Geometry: final body of the model. Coordinates: model frame, mm. Face numbers are marked on the shaded views. A direction names the side the tool comes from. Give positions to 0.01 mm unless a question says otherwise; leave off trailing zeros. Order: outer loops, then holes, each group sorted by start corner. A loop starts at its lowest first (then second) coordinate and runs counter-clockwise, first axis right, second up. Notation, with made-up numbers: (-38, 46.5) -> (21, 46.5) arc R15 cw to (21, 55.5) -> close; hole circle Ø1 at (76, 51.25). An arc over 180 degrees is marked (long way). Write item = value, one per line.
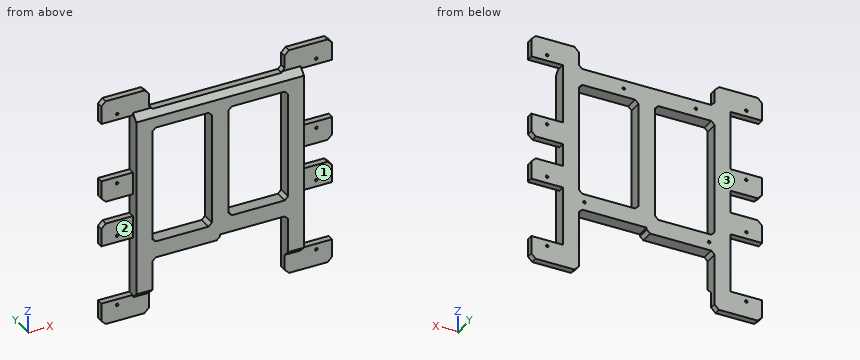
```python
from build123d import *

# Parameters (mm, degrees)
SKETCH1_W               = 89.4
SKETCH1_H               = 89.4
SKETCH1_R               = 0.5
BOSS_EXTRUDE1_DEPTH     = 2.5
SKETCH5_W               = 65
SKETCH5_H               = 74
BOSS_EXTRUDE3_DEPTH     = 2.5
SKETCH7_R               = 0.5
CUT_EXTRUDE2_DEPTH      = 4
CUT_EXTRUDE1_DEPTH      = 64.412774738
CUT_EXTRUDE1_DEPTH_BACK = 64.412774738
SKETCH2_W               = 12.2
SKETCH2_H               = 23
SKETCH2_W_2             = 52.6
SKETCH2_H_2             = 8.025
SKETCH2_W_3             = 23.1
SKETCH2_H_3             = 45.67
SKETCH2_H_4             = 43.68
SKETCH2_H_5             = 8.8
CHAMFER2_SIZE           = 1.3
CHAMFER3_SIZE           = 1.3
CHAMFER4_SIZE           = 1.7
CHAMFER5_SIZE           = 2.5


with BuildPart() as part:
    # Sketch1 → Boss-Extrude1 (new body)
    with BuildSketch(Plane(origin=(0, 0, 0), x_dir=(1, 0, 0), z_dir=(0, 1, 0))):
        Rectangle(SKETCH1_W, SKETCH1_H)
        with Locations(Location((-38.6, 38.3, 0), (0, 0, 270))):
            Circle(SKETCH1_R, mode=Mode.SUBTRACT)
        with Locations(Location((-38.6, 10.5, 0), (0, 0, 270))):
            Circle(SKETCH1_R, mode=Mode.SUBTRACT)
        with Locations(Location((-38.6, -10.5, 0), (0, 0, 270))):
            Circle(SKETCH1_R, mode=Mode.SUBTRACT)
        with Locations(Location((-38.6, -38.3, 0), (0, 0, 270))):
            Circle(SKETCH1_R, mode=Mode.SUBTRACT)
        with Locations(Location((38.6, -38.3, 0), (0, 0, 90))):
            Circle(SKETCH1_R, mode=Mode.SUBTRACT)
        with Locations(Location((38.6, -10.5, 0), (0, 0, 90))):
            Circle(SKETCH1_R, mode=Mode.SUBTRACT)
        with Locations(Location((38.6, 10.5, 0), (0, 0, 90))):
            Circle(SKETCH1_R, mode=Mode.SUBTRACT)
        with Locations(Location((38.6, 38.3, 0), (0, 0, 90))):
            Circle(SKETCH1_R, mode=Mode.SUBTRACT)
    extrude(amount=BOSS_EXTRUDE1_DEPTH)

    # Sketch5 → Boss-Extrude3 (add)
    with BuildSketch(Plane.XZ):
        Rectangle(SKETCH5_W, SKETCH5_H)
    extrude(amount=BOSS_EXTRUDE3_DEPTH)

    # Sketch7 → Cut-Extrude2 (cut)
    with BuildSketch(Plane(origin=(0, 2.5, 0), x_dir=(1, 0, 0), z_dir=(0, 1, 0))):
        with Locations(Location((-24.15, 18.595, 0), (0, 0, 270))):
            Circle(SKETCH7_R)
        with Locations(Location((24.15, 16.605, 0), (0, 0, 270))):
            Circle(SKETCH7_R)
        with Locations(Location((-19.07, -33.475, 0), (0, 0, 270))):
            Circle(SKETCH7_R)
        with Locations(Location((8.86, -33.475, 0), (0, 0, 270))):
            Circle(SKETCH7_R)
    extrude(amount=-CUT_EXTRUDE2_DEPTH, mode=Mode.SUBTRACT)

    # Sketch2 → Cut-Extrude1 (cut, two sides: drawn at the far end of the back side and taken through both)
    with BuildSketch(Plane(origin=(0, 2.5, 0), x_dir=(1, 0, 0), z_dir=(0, 1, 0)).offset(-CUT_EXTRUDE1_DEPTH_BACK)):
        with Locations((-38.6, 24.55)):
            Rectangle(SKETCH2_W, SKETCH2_H)
        Polygon((-26.3, 44.7), (26.3, 44.7), (26.3, 24.23), (26.3, 19.805), (0, 19.805), (0, 21.795), (-26.3, 21.795), align=None)
        with Locations((0, -40.6875)):
            Rectangle(SKETCH2_W_2, SKETCH2_H_2)
        with Locations((-14.75, -7.44)):
            Rectangle(SKETCH2_W_3, SKETCH2_H_3)
        with Locations((14.75, -8.435)):
            Rectangle(SKETCH2_W_3, SKETCH2_H_4)
        with Locations((-38.6, 0)):
            Rectangle(SKETCH2_W, SKETCH2_H_5)
        with Locations((38.6, 0)):
            Rectangle(SKETCH2_W, SKETCH2_H_5)
        with Locations((38.6, 24.55)):
            Rectangle(SKETCH2_W, SKETCH2_H)
        with Locations((38.6, -24.55)):
            Rectangle(SKETCH2_W, SKETCH2_H)
        with Locations((-38.6, -24.55)):
            Rectangle(SKETCH2_W, SKETCH2_H)
    extrude(amount=CUT_EXTRUDE1_DEPTH + CUT_EXTRUDE1_DEPTH_BACK, mode=Mode.SUBTRACT)

    # Chamfer2
    chamfer2_edges = [part.edges().sort_by_distance(p)[0] for p in [
        (0, 0, -21.795),
    ]]
    chamfer(chamfer2_edges, length=CHAMFER2_SIZE)

    # Chamfer3
    chamfer3_edges = [part.edges().sort_by_distance(p)[0] for p in [
        (-26.3, 0, -21.795),
        (26.3, 0, 36.675),
        (-26.3, 0, 36.675),
        (-26.3, 0, 30.275),
        (-3.2, 0, 30.275),
        (3.2, 0, 30.275),
        (26.3, 0, 30.275),
        (-3.2, 0, -15.395),
        (3.2, 0, -13.405),
        (26.3, 0, -13.405),
        (26.3, 0, -19.805),
        (-26.3, 0, -15.395),
    ]]
    chamfer(chamfer3_edges, length=CHAMFER3_SIZE)

    # Chamfer4
    chamfer4_edges = [part.edges().sort_by_distance(p)[0] for p in [
        (26.3, 1.25, 44.7),
        (-26.3, 1.25, 44.7),
        (-44.7, 1.25, 4.4),
        (-44.7, 1.25, -4.4),
        (-26.3, 1.25, -44.7),
        (26.3, 1.25, -44.7),
        (44.7, 1.25, -4.4),
        (44.7, 1.25, 4.4),
        (-44.7, 1.25, -44.7),
        (44.7, 1.25, -44.7),
        (44.7, 1.25, 44.7),
        (-44.7, 1.25, 44.7),
    ]]
    chamfer(chamfer4_edges, length=CHAMFER4_SIZE)

    # Chamfer5
    chamfer5_edges = [part.edges().sort_by_distance(p)[0] for p in [
        (28.9125, -2.5, 37),
        (29.4, -2.5, -37),
        (-29.4, -2.5, -37),
    ]]
    chamfer(chamfer5_edges, length=CHAMFER5_SIZE - 0.0001)  # a hair under: the kernel refuses the full size


solid = part.part
```
1) First-contact query: P1, Ø3, axis at y = 1.5, z = -32, coming from the +X side; P2, Ø2.5, axis at y = -0.5, z = -3.5, coming from the +X side; P3, Ø3, axis at y = 0.5, z = 4, coming from the -X side. Flat tips, straight axial feed; report the tip coordinate or a pass-through.
Check sheet entries:
P1 = 32.5
P2 = 43.25
P3 = -44.1
2) Section query D-D (z = -30). Output: boundary loops of the cut face in (x, y).
Check sheet entries:
outline = (-32.5, -2.5) -> (-26.3, -2.5) -> (-26.3, 2.5) -> (-32.5, 2.5) -> close; (26.3, -2.5) -> (32.5, -2.5) -> (32.5, 2.5) -> (26.3, 2.5) -> close
3) Section query C-C (x = -34.5). Output: boundary loops of the cut face in (y, z), plus the area to 3 significant figures.
Check sheet entries:
outline = (0, -44.7) -> (2.5, -44.7) -> (2.5, -36.05) -> (0, -36.05) -> close; (0, -13.05) -> (2.5, -13.05) -> (2.5, -4.4) -> (0, -4.4) -> close; (0, 4.4) -> (2.5, 4.4) -> (2.5, 13.05) -> (0, 13.05) -> close; (0, 36.05) -> (2.5, 36.05) -> (2.5, 44.7) -> (0, 44.7) -> close
area = 86.5 mm²
4) Line query: line 1 (X direction, y = 1.3, z = 38.3); line 2 (X direction, y = 1.05, z = 28.5); line 3 (Z direction, x = 40.5, y = 0.2). Output: solid intervals per line, ascending. Write a range as from..to.
Check sheet entries:
line_1 = -44.7..-39.1, -38.1..-26.3, 26.3..38.1, 39.1..44.7
line_2 = -32.5..-26.3, -3.2..3.2, 26.3..32.5
line_3 = -44.7..-36.05, -13.05..-4.4, 4.4..13.05, 36.05..44.7
5) Reachability of the marked faces 1, 2 and 3 from +Z, -Z, +X, -X, +Y, -Y: full face, straight path, thin tool, end or side. Return the list, or none.
Check sheet entries:
face_1 = +Z, -Z, +X, -Y
face_2 = +Z, -Z, -X, -Y
face_3 = +Z, -Z, +X, -X, +Y
6) Section query B-B (z = 0). Output: boundary loops of the cut face in (x, y).
Check sheet entries:
outline = (-32.5, -2.5) -> (-26.3, -2.5) -> (-26.3, 2.5) -> (-32.5, 2.5) -> close; (-3.2, -2.5) -> (3.2, -2.5) -> (3.2, 2.5) -> (-3.2, 2.5) -> close; (26.3, -2.5) -> (32.5, -2.5) -> (32.5, 2.5) -> (26.3, 2.5) -> close
7) Section query A-A (x = 7). Output: boundary loops of the cut face in (y, z) (3 decimals).
Check sheet entries:
outline = (-2.5, -19.805) -> (2.5, -19.805) -> (2.5, -13.405) -> (-2.5, -13.405) -> close; (-2.5, 30.275) -> (2.5, 30.275) -> (2.5, 36.675) -> (-0.325, 36.675) -> (-2.5, 34.5) -> close
